Verification items for the finished model (mm, model axes). Face numbers are marked on the shaded views. A direction names the side the tool comes from. Coordinates: 2 decimals unless noted, no trailing zeros. Loops run counter-clockwise (first coordinate to the right, second up) from the corner with the lowest first, then second, coordinate; pieces in that order, holes last.
Q1. Sectioned sample at C-C (x = -33.5). Enter the section's corners in (y, z), then the cut area to 3 significant figures.
Q2. Sectioned sample at A-A (y = -17.75). Enter the section's corners in (x, z).
Q3. Go/stop test with flat-tipped pins: P1, Ø2, axis at x = -24.5, y = -16, coming from the -Z side; P2, Ø5, axis at x = 30, y = -14, coming from the -Z side; P3, Ø6, axis at y = -11, z = 27, coming from the +X side; P4, Ø5, axis at x = -29.5, z = -26, coming from the +Y side. Record where each tip stops, or that it passes through.
Q4. Sectioned sample at D-D (x = -5.5). Enter the section's corners in (y, z).
Q5. Access from +Z, -Z, +X, -X, +Y, -Y to the whole of each face (thin tool, end or side, straight path). Record for the marked faces 1, 2 and 3.
Q6. Material ranges on probe 1 along X at (y, z) = (-20.75, -46.5); probe 2 along X at (y, z) = (-20.75, -17.5); probe 3 along Z at (x, y) = (-16, -10.25), recorded low to high.
Q7. Mould release check, pull along Z, two halves, no side actions. Record for the marked faces 4, 5 and 6: +Z half, -Z half, draft (parallel to the pull), parting line (faces both ways), or undercut.
Q8. Sectioned sample at B-B (z = -28.5). Enter the section's corners in (x, y), then the cut area to 3 significant figures.
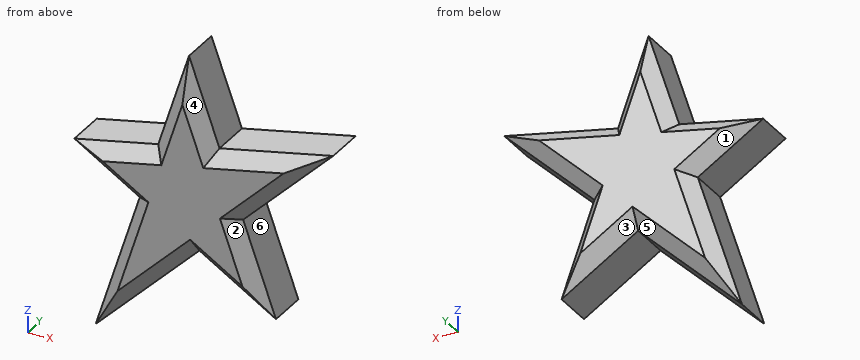
```python
from build123d import *

# Parameters (mm, degrees)
F1_DEPTH = 25.4
F2_SIZE  = 5.08
F3_SIZE  = 5.08


with BuildPart() as f1:
    # F0 (on Front) → F1 (new body)
    with BuildSketch(Plane.XZ):
        Polygon((3.910511, -15.808209), (32.639593, -33.872131), (20.304644, 0.264795), (54.112185, 33.410113), (11.456304, 24.752544), (0, 56.457825), (-11.533625, 20.086437), (-43.014806, 13.69692), (-18.456406, -1.744611), (-35.019126, -53.975292), align=None)
    extrude(amount=F1_DEPTH)

    # F2
    f2_edges = [f1.edges().sort_by_distance(p)[0] for p in [
        (-5.766813, -25.4, 38.272131),
        (-27.274216, -25.4, 16.891679),
        (-15.554307, -25.4, -34.89175),
        (18.275052, -25.4, -24.84017),
        (26.472118, -25.4, -16.803668),
        (37.208414, -25.4, 16.837454),
        (32.784244, -25.4, 29.081329),
        (5.728152, -25.4, 40.605185),
        (-30.735606, -25.4, 5.976154),
        (-26.737766, -25.4, -27.859951),
    ]]
    chamfer(f2_edges, length=F2_SIZE)

    # F3
    f3_edges = [f1.edges().sort_by_distance(p)[0] for p in [
        (-15.554307, 0, -34.89175),
        (18.275052, 0, -24.84017),
        (26.472118, 0, -16.803668),
        (37.208414, 0, 16.837454),
        (32.784244, 0, 29.081329),
        (5.728152, 0, 40.605185),
        (-5.766813, 0, 38.272131),
        (-27.274216, 0, 16.891679),
        (-30.735606, 0, 5.976154),
        (-26.737766, 0, -27.859951),
    ]]
    chamfer(f3_edges, length=F3_SIZE)


solid = f1.part
```
Geometry check:
1. outline: (-23.91, 11.96) - (-20.32, 7.71) - (-5.08, 7.71) - (-1.49, 11.96) - (-5.08, 15.63) - (-20.32, 15.63) - close; (-21.02, -51.5) - (-20.32, -52.49) - (-5.08, -52.49) - (-4.38, -51.5) - (-5.08, -49.18) - (-20.32, -49.18) - close
1. area: 202 mm2
2. outline: (-43.01, 13.7) - (-18.46, -1.74) - (-35.02, -53.98) - (3.91, -15.81) - (32.64, -33.87) - (20.3, 0.26) - (54.11, 33.41) - (11.46, 24.75) - (0, 56.46) - (-11.53, 20.09) - close
3. P1: stops at z = -44.64
3. P2: stops at z = -33.78
3. P3: stops at x = 50.63
3. P4: passes through
4. outline: (-25.4, -17.92) - (-20.32, -25.03) - (-5.08, -25.03) - (0, -17.92) - (0, 22.31) - (-5.08, 39.11) - (-20.32, 39.11) - (-25.4, 22.31) - close
5. face 1: -X, +Y
5. face 2: +X, -Y
5. face 3: -Z, +Y
6. probe 1: x = -32.2 to -28.01
6. probe 2: x = -23 to 1.57, 7.41 to 26.27
6. probe 3: z = -35.33 to 19.18
7. face 4: +Z half
7. face 5: -Z half
7. face 6: undercut
8. outline: (-26.94, -20.32) - (-21.61, -25.4) - (-16.29, -25.4) - (-9.03, -20.32) - (-9.03, -5.08) - (-16.29, 0) - (-21.61, 0) - (-26.94, -5.08) - close; (24.1, -20.32) - (28.31, -22.56) - (30.7, -20.32) - (30.7, -5.08) - (28.31, -2.84) - (24.1, -5.08) - close
8. area: 506 mm2
